from build123d import *

# Parameters (mm, degrees)
BOSS_EXTRU_1_DEPTH      = 1.6
ESQUISSE5_R             = 2
ENL_V_MAT_EXTRU_1_DEPTH = 1.6
ECRAN_W                 = 77.498087901
ECRAN_H                 = 56.00411385
BOSS_EXTRU_2_DEPTH      = 3
ECRAN_NOIR_W            = 70.00084158
ECRAN_NOIR_H            = 51.004481936
ENL_V_MAT_EXTRU_2_DEPTH = 0.5
NAPPE_CONTACTEURS_W     = 5.000690241
NAPPE_CONTACTEURS_H     = 39.972572183
ENL_V_MAT_EXTRU_3_DEPTH = 0.5
CONG_1_R                = 0.5


with BuildPart() as part:
    # Esquisse1 → Boss.-Extru.1 (new body)
    with BuildSketch(Plane(origin=(0, 0, 0), x_dir=(1, 0, 0), z_dir=(0, 1, 0))):
        Polygon((0, 0), (83.3, 0), (83.3, 74), (75, 74), (75, 80), (57.3, 80), (57.3, 85), (0, 85), align=None)
    extrude(amount=BOSS_EXTRU_1_DEPTH)

    # Esquisse5 → Enlèv. mat.-Extru.1 (cut)
    with BuildSketch(Plane(origin=(0, 1.6, 0), x_dir=(1, 0, 0), z_dir=(0, 1, 0))):
        with Locations(Location((54.3, 82, 0), (0, 0, 270))):
            Circle(ESQUISSE5_R)
        with Locations(Location((3, 82, 0), (0, 0, 270))):
            Circle(ESQUISSE5_R)
        with Locations(Location((3, 2.996959755, 0), (0, 0, 270))):
            Circle(ESQUISSE5_R)
        with Locations(Location((80.298286248, 2.996959755, 0), (0, 0, 270))):
            Circle(ESQUISSE5_R)
    extrude(amount=-ENL_V_MAT_EXTRU_1_DEPTH, mode=Mode.SUBTRACT)

    # ecran → Boss.-Extru.2 (add)
    with BuildSketch(Plane(origin=(0, 1.6, 0), x_dir=(1, 0, 0), z_dir=(0, 1, 0))):
        with Locations((44.55095605, 45.806316508)):
            Rectangle(ECRAN_W, ECRAN_H)
    extrude(amount=BOSS_EXTRU_2_DEPTH)

    # ecran noir → Enlèv. mat.-Extru.2 (cut)
    with BuildSketch(Plane(origin=(0, 4.6, 0), x_dir=(1, 0, 0), z_dir=(0, 1, 0))):
        with Locations((43.298888969, 45.808865656)):
            Rectangle(ECRAN_NOIR_W, ECRAN_NOIR_H)
    extrude(amount=-ENL_V_MAT_EXTRU_2_DEPTH, mode=Mode.SUBTRACT)

    # nappe contacteurs → Enlèv. mat.-Extru.3 (cut)
    with BuildSketch(Plane(origin=(0, 4.6, 0), x_dir=(1, 0, 0), z_dir=(0, 1, 0))):
        with Locations((80.79965488, 48.80952599)):
            Rectangle(NAPPE_CONTACTEURS_W, NAPPE_CONTACTEURS_H)
    extrude(amount=-ENL_V_MAT_EXTRU_3_DEPTH, mode=Mode.SUBTRACT)

    # Congé1
    cong_1_edges = [part.edges().sort_by_distance(p)[0] for p in [
        (83.3, 4.1, -48.809525991),
    ]]
    fillet(cong_1_edges, radius=CONG_1_R)


solid = part.part
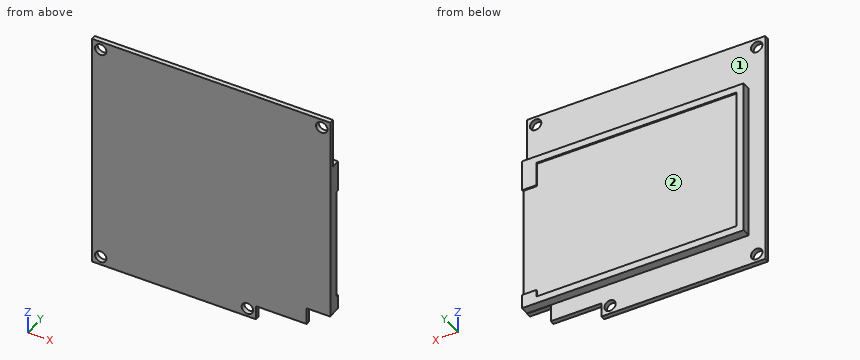
Work out the finished part from the listing and answer in its coordinate system (mm). Face numbers are marked on the shaded views. Coordinates: 2 decimals unless noted, no trailing zeros. Write each loop counter-clockwise with the first axis right and the second up, starting at its lowest first coordinate (ties: lowest second). Pieces come first, ordered by that corner, then holes. Notation, with made-up numbers: (2, 68) - (51, 68) arc R31 ccw to (51, 99) - close; hole circle Ø10 at (-23.75, 12). An arc over 180 degrees is marked (long way). One line per question, with ' | ' between items.
1) Consider probe 1 along X at (y, z) = (1.25, -82); probe 2 along Y at (x, z) = (68, -71); probe 3 along Z at (x, y) = (66.5, 1.95). Determine where each line is inside the solid, lowest interval first. Write a range as [from, to].
Checks:
probe 1: [0, 1], [5, 52.3], [56.3, 57.3] | probe 2: [0, 4.1] | probe 3: [-73.81, -17.8]
2) Find section D-D, the plane z = -51. Determine the outline of the cut face in (x, y).
Checks:
outline: (0, 0) - (83.3, 0) - (83.3, 3.6) arc R0.5 ccw to (82.8, 4.1) - (8.3, 4.1) - (8.3, 4.6) - (5.8, 4.6) - (5.8, 1.6) - (0, 1.6) - close
3) Find section A-A, the plane x = 3. Determine the outline of the cut face in (y, z).
Checks:
outline: (0, -85) - (1.6, -85) - (1.6, -84) - (0, -84) - close; (0, -80) - (1.6, -80) - (1.6, -5) - (0, -5) - close; (0, -1) - (1.6, -1) - (1.6, 0) - (0, 0) - close
4) The mould has two halves that part along Z. Classify the marked faces 1 and 2: +Z half, -Z half, draft (parallel to the pull), parting line (faces both ways), or undercut.
Checks:
face 1: draft | face 2: undercut
5) Find section B-B, the plane x = 54.3. Determine the outline of the cut face in (y, z).
Checks:
outline: (0, -85) - (1.6, -85) - (1.6, -84) - (0, -84) - close; (0, -80) - (1.6, -80) - (1.6, -73.81) - (4.6, -73.81) - (4.6, -71.31) - (4.1, -71.31) - (4.1, -20.31) - (4.6, -20.31) - (4.6, -17.8) - (1.6, -17.8) - (1.6, 0) - (0, 0) - close
6) Find section C-C, the plane z = -82. Determine the outline of the cut face in (x, y).
Checks:
outline: (0, 0) - (1, 0) - (1, 1.6) - (0, 1.6) - close; (5, 0) - (52.3, 0) - (52.3, 1.6) - (5, 1.6) - close; (56.3, 0) - (57.3, 0) - (57.3, 1.6) - (56.3, 1.6) - close
7) Flat-ended cylindrical pins translate along their axes: P1, Ø0.8, axis at x = 81, y = 4, coming from the -Z side; P2, Ø1.3, axis at y = 0.5, z = -76.5, coming from the +X side; P3, Ø2.5, axis at y = 3.5, z = -44, coming from the -X side. Find the tip coordinate at first contact, or state that the pin passes through.
Checks:
P1: z = -73.81 | P2: x = 75 | P3: x = 5.8
